Autodesk Fusion 360 part; units mm, degrees
sketch "Sketch1" plane through (0, 0, 0) normal (0, 0, 1) x (1, 0, 0)
  circle A0 centre (0, 0) radius 7.5
  circle A1 centre (0, 0) radius 9.7
  circle A2 centre (11.7, 0) radius 2
  circle A3 centre (11.7, 0) radius 4.2
  line L0 (-19.1275, 0) -> (19.1275, 0) construction
  line L1 (0, 53.4087) -> (0, -53.4087) construction
  circle A4 centre (9.1606, -1.7781) radius 1.1
  circle A5 centre (14.2394, -1.7781) radius 1.1
  circle A6 centre (7.4478, 4.3) radius 1.1
  line L2 (0, 0) -> (7.4478, 4.3) construction
  line L3 (0, 0) -> (11.7, 0) construction
  line L4 (9.1606, -1.7781) -> (11.7, 0) construction
  line L5 (14.2394, -1.7781) -> (11.7, 0) construction
  line L6 (9.1606, -1.7781) -> (14.2394, -1.7781) construction
  dimension "d5_1_1_2_1_1" = 15
  dimension "d6_1_1_2_1_1" = 2.2
  dimension "d7_1_1_2_1_1" = 4
  dimension "d9_1_1_2_1_1" = 2.2
  dimension "d17_1_1_2_1_1" = 2.2
  dimension "d18_1_1_2_1_1" = 2.2
  dimension "d23_1_1_2_1_1" = 2.2
  dimension "d32_1_1" = 110
  dimension "d34_1_1" = 90
  dimension "d36_1" = 30
  dimension "d47" = 5.0787
extrude "Extrude1" add sketch "Sketch1" along normal blind 5 contours A0 A1 A3 A6 | A1 A3 A4 | A6 | A1 A2 A3 A5 | A1 A3 A4 | A1 A4 | A1 A2 A4 | A1 A4 | A5 picked at (6.1986, 5.9178)
fillet "Fillet1" radius 0.5 1 edges at (9.2647, -2.8732, 2.5)
chamfer "Chamfer2" distance 0.6 angle 45 16 edges at (7.9978, 3.3474, 5) (-9.6544, -0.9396, 5) (9.3007, -2.9443, 5) (10.2033, -2.1285, 5) (11.7, 2, 5) (13.6084, -2.6792, 5) (12.963, 4.0056, 5) (-7.2444, -1.9411, 5) (10.2033, -2.1285, 0) (11.7, 2, 0) (13.6084, -2.6792, 0) (12.963, 4.0056, 0) (-7.2444, -1.9411, 0) (7.9978, 3.3474, 0) (-9.6544, -0.9396, 0) (9.3007, -2.9443, 0)
equation "d6_1_1_2_1_1 = ClipWall"
equation "d9_1_1_2_1_1 = ClipWall"
equation "d17_1_1_2_1_1 = ClipWall"
equation "d18_1_1_2_1_1 = ClipWall"
equation "d21_1_1_2_1_1 = Thickness"
equation "d23_1_1_2_1_1 = ClipWall"
equation "ClipWall = 2.2 mm"
equation "Thickness = 5 mm"
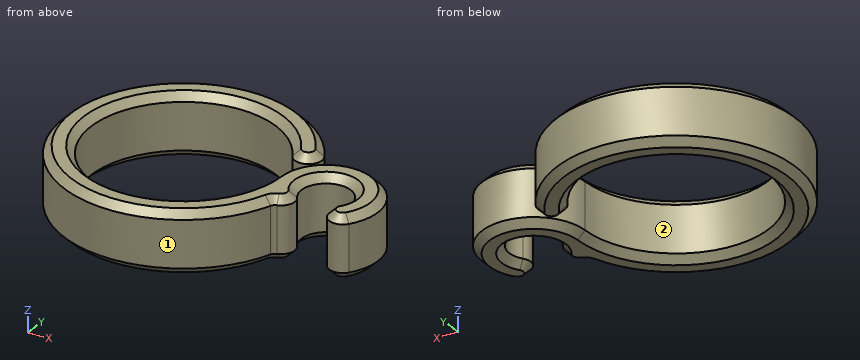
Here's how the part is built. I have some questions about the finished solid (model axes, mm). Face numbers are marked on the shaded views. Coordinates: 2 decimals unless noted, no trailing zeros. Write each loop counter-clockwise with the first axis right and the second up, starting at its lowest first coordinate (ties: lowest second). Pieces come first, ordered by that corner, then holes. Notation, with made-up numbers: (31, 4.5) - (63, 4.5) arc R14 cw to (63, 20.5) - close; hole circle Ø1 at (33, -30.75). An arc over 180 degrees is marked (long way). One line per item, written item: value.
1) Suppose I cut it at A-A on y = 0. Write out the boundary of the cut face in (x, z).
Model answer:
outline: (-9.7, 0.6) - (-9.1, 0) - (-8.1, 0) - (-7.5, 0.6) - (-7.5, 4.4) - (-8.1, 5) - (-9.1, 5) - (-9.7, 4.4) - close; (7.5, 0.6) - (8.1, 0) - (9.1, 0) - (9.7, 0.6) - (9.7, 4.4) - (9.1, 5) - (8.1, 5) - (7.5, 4.4) - close; (13.7, 0.6) - (14.3, 0) - (15.3, 0) - (15.9, 0.6) - (15.9, 4.4) - (15.3, 5) - (14.3, 5) - (13.7, 4.4) - close
2) Suppose I cut it at C-C on x = 11.7. Write out the boundary of the cut face in (y, z), and give its area (3 significant figures).
Model answer:
outline: (2, 0.6) - (2.6, 0) - (3.6, 0) - (4.2, 0.6) - (4.2, 4.4) - (3.6, 5) - (2.6, 5) - (2, 4.4) - close
area: 10.3 mm²
3) We'd pull the mould along X, two halves only. Please class the marked faces 1 and 2: pulls with the +X half, pulls with the -X half, needs draft (parallel to the pull), parting line crosses it, or undercut.
Model answer:
face 1: parting line crosses it
face 2: undercut
4) I'm going to push flat-ended pins straight in: P1, Ø3, axis at x = 1.5, y = -4, coming from the -Z side; P2, Ø2, axis at y = -7, z = 4, coming from the +X side; P3, Ø6, axis at x = -6.5, y = 7, coming from the -Z side; P4, Ø1.5, axis at x = 2.5, z = 1, coming from the -Y side. Where does each tip first touch, or does it pass through?
Model answer:
P1: passes through
P2: stops at x = 7.62
P3: stops at z = 0
P4: stops at y = -9.54
5) Suppose I cut it at B-B on x = 0. Write out the boundary of the cut face in (y, z).
Model answer:
outline: (-9.7, 0.6) - (-9.1, 0) - (-8.1, 0) - (-7.5, 0.6) - (-7.5, 4.4) - (-8.1, 5) - (-9.1, 5) - (-9.7, 4.4) - close; (7.5, 0.6) - (8.1, 0) - (9.1, 0) - (9.7, 0.6) - (9.7, 4.4) - (9.1, 5) - (8.1, 5) - (7.5, 4.4) - close
6) I need wall thicknesses on line 1 along X through (y, z) = (0, 3.5); line 2 along Y through (x, z) = (0, 3.6); line 3 along X through (y, z) = (-2.75, 3.55). Which ranges of each line are inside material? Lowest first, please.
Model answer:
line 1: x = -9.7 to -7.5, 7.5 to 9.7, 13.7 to 15.9
line 2: y = -9.7 to -7.5, 7.5 to 9.7
line 3: x = -9.3 to -6.98, 6.98 to 9.68, 13.72 to 14.75
